Verification items for the finished model (mm, model axes). Face numbers are marked on the shaded views. Round coordinates to 2 decimals unless told otherwise and drop trailing zeros. Loops run counter-clockwise (first coordinate to the right, second up) from the corner with the lowest first, then second, coordinate; pieces in that order, holes last. Notation, with made-up numbers: (-25.5, 61.25) -> (-3.5, 61.25) arc R27 ccw to (-3.5, 81.25) -> close; hole circle Ø9 at (-8.5, 3). An arc over 180 degrees is marked (long way). Write item = value, one per line.
```python
from build123d import *

# Parameters (mm, degrees)
F0_R     = 50
F0_R_2   = 3
F1_DEPTH = 15
F3_D     = 5.1
F4_R     = 39
F5_DEPTH = 2


with BuildPart() as f1:
    # F0 (on Front) → F1 (new body)
    with BuildSketch(Plane.XZ):
        Circle(F0_R)
        Circle(F0_R_2, mode=Mode.SUBTRACT)
    extrude(amount=-F1_DEPTH)

    # F3 (through all)
    with Locations(Plane.XZ):
        with Locations((-22.5, 38.971143), (22.5, 38.971143), (45, 0), (22.5, -38.971143), (-22.5, -38.971143), (-45, 0)):
            Hole(F3_D / 2)

    # F4 (on Front) → F5 (cut)
    with BuildSketch(Plane.XZ):
        Circle(F4_R)
    extrude(amount=-F5_DEPTH, mode=Mode.SUBTRACT)


solid = f1.part
```
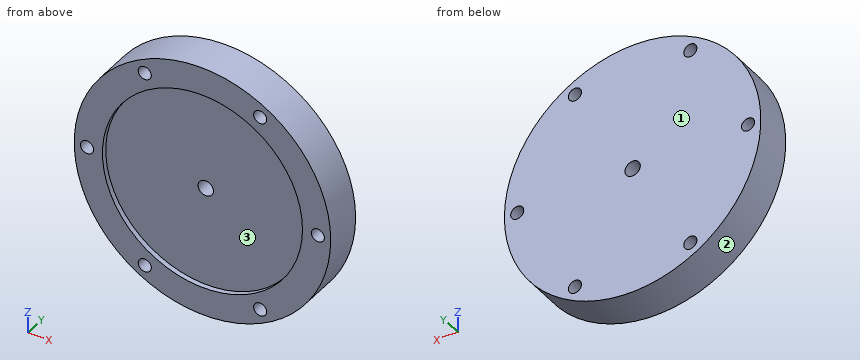
(1) Sectioned sample at B-B, the plane x = 0. Record the cut outline in (y, z).
Filled sheet:
outline = (0, -50) -> (15, -50) -> (15, -3) -> (2, -3) -> (2, -39) -> (0, -39) -> close; (0, 39) -> (2, 39) -> (2, 3) -> (15, 3) -> (15, 50) -> (0, 50) -> close
(2) Go/stop test with flat-tipped pins: pin 1 Ø6 at (y, z) = (2.5, -4) entering from -X; pin 2 Ø6.5 at (x, z) = (-45, 0) entering from +Y; pin 3 Ø1 at (x, y) = (-0.5, 1.5) entering from +Z; pin 4 Ø4 at (x, y) = (-26, 12) entering from +Z. Record where each tip stops, or that it passes through.
Filled sheet:
pin_1 = -49.99
pin_2 = 15
pin_3 = 50
pin_4 = 43.86
(3) Sectioned sample at D-D, the plane y = 13.5. Record the cut outline in (x, z), and give its area (3 significant figures).
Filled sheet:
outline = circle Ø100 at (0, 0); hole circle Ø5.1 at (-45, 0); hole circle Ø5.1 at (-22.5, -38.97); hole circle Ø5.1 at (-22.5, 38.97); hole circle Ø6 at (0, 0); hole circle Ø5.1 at (22.5, -38.97); hole circle Ø5.1 at (22.5, 38.97); hole circle Ø5.1 at (45, 0)
area = 7,700 mm2
(4) Draft check along Z on the marked faces 1, 2 and 3. Enter one of: released by +Z, released by -Z, zero draft, split by the parting line, or undercut.
Filled sheet:
face_1 = zero draft
face_2 = split by the parting line
face_3 = undercut
(5) Material ranges on probe 1 along X at (y, z) = (5.25, 37.5); probe 2 along Z at (x, y) = (-22.5, 10.5); probe 3 along Z at (x, y) = (-22, 13), recorded low to high. Write a range as from..to.
Filled sheet:
probe_1 = -33.07..-24.58, -20.42..20.42, 24.58..33.07
probe_2 = -44.65..-41.52, -36.42..36.42, 41.52..44.65
probe_3 = -44.9..-41.47, -36.47..36.47, 41.47..44.9
(6) Sectioned sample at A-A, the plane z = 0. Record the cut outline in (x, y).
Filled sheet:
outline = (-50, 0) -> (-47.55, 0) -> (-47.55, 15) -> (-50, 15) -> close; (-42.45, 0) -> (-39, 0) -> (-39, 2) -> (-3, 2) -> (-3, 15) -> (-42.45, 15) -> close; (3, 2) -> (39, 2) -> (39, 0) -> (42.45, 0) -> (42.45, 15) -> (3, 15) -> close; (47.55, 0) -> (50, 0) -> (50, 15) -> (47.55, 15) -> close
(7) Sectioned sample at C-C, the plane x = 22.5. Record the cut outline in (y, z).
Filled sheet:
outline = (0, -44.65) -> (15, -44.65) -> (15, -41.52) -> (0, -41.52) -> close; (0, -36.42) -> (15, -36.42) -> (15, 36.42) -> (0, 36.42) -> (0, 31.86) -> (2, 31.86) -> (2, -31.86) -> (0, -31.86) -> close; (0, 41.52) -> (15, 41.52) -> (15, 44.65) -> (0, 44.65) -> close
